Part model, mm, in its own coordinate system. Face numbers are marked on the shaded views. A direction names the side the tool comes from. Give positions to 0.01 mm unless a question says otherwise; leave off trailing zeros. Order: outer loops, then holes, each group sorted by start corner. A loop starts at its lowest first (then second) coordinate and runs counter-clockwise, first axis right, second up. Notation, with made-up numbers: (-33, -35) - (-27, -35) arc R27 cw to (-27, -3) - close; hole circle Ø2 at (-29.75, 15). An arc over 180 degrees is marked (long way). Use a Markdown table: item, result. Add a question column.
from build123d import *

# Parameters (mm, degrees)
SKETCH1_W           = 15.875
SKETCH1_H           = 44.45
BASE_EXTRUDE_DEPTH  = 22.225
SKETCH2_W           = 26.98496
SKETCH2_H           = 26.98496
BOSS_EXTRUDE1_DEPTH = 59.39536
SKETCH3_W           = 38.1
SKETCH3_H           = 38.1
BOSS_EXTRUDE2_DEPTH = 15.875
SKETCH4_R           = 2.09296
BOSS_EXTRUDE3_DEPTH = 59.39536
SKETCH5_R           = 1.45796
CUT_EXTRUDE1_DEPTH  = 75.27036
SKETCH6_R           = 4.7625
CUT_EXTRUDE2_DEPTH  = 75.27036
SKETCH8_R           = 3.175
CUT_EXTRUDE3_DEPTH  = 6.35


with BuildPart() as part:
    # Sketch1 → Base-Extrude (new, symmetric)
    with BuildSketch(Plane.XY):
        Rectangle(SKETCH1_W, SKETCH1_H)
    extrude(amount=BASE_EXTRUDE_DEPTH, both=True)

    # Sketch2 → Boss-Extrude1 (add)
    with BuildSketch(Plane(origin=(7.9375, 0, 0), x_dir=(0, 0, -1), z_dir=(1, 0, 0))):
        Rectangle(SKETCH2_W, SKETCH2_H)
    extrude(amount=BOSS_EXTRUDE1_DEPTH)

    # Sketch3 → Boss-Extrude2 (add)
    with BuildSketch(Plane(origin=(67.33286, -2.916482086, 3.369055623), x_dir=(0, 0, -1), z_dir=(1, 0, 0))):
        with Locations((3.369055623, 2.916482086)):
            Rectangle(SKETCH3_W, SKETCH3_H)
    extrude(amount=BOSS_EXTRUDE2_DEPTH)

    # Sketch4 → Boss-Extrude3 (add)
    with BuildSketch(Plane(origin=(7.9375, 0, 0), x_dir=(0, 0, -1), z_dir=(1, 0, 0))):
        with Locations((-13.49248, 13.49248)):
            Circle(SKETCH4_R)
        with Locations((-13.49248, -13.49248)):
            Circle(SKETCH4_R)
        with Locations((13.49248, 13.49248)):
            Circle(SKETCH4_R)
        with Locations((13.49248, -13.49248)):
            Circle(SKETCH4_R)
    extrude(amount=BOSS_EXTRUDE3_DEPTH)

    # Sketch5 → Cut-Extrude1 (cut)
    with BuildSketch(Plane(origin=(83.20786, 0, 0), x_dir=(0, 0, -1), z_dir=(1, 0, 0))):
        with Locations((-13.49248, 13.49248)):
            Circle(SKETCH5_R)
        with Locations((-13.49248, -13.49248)):
            Circle(SKETCH5_R)
        with Locations((13.49248, 13.49248)):
            Circle(SKETCH5_R)
        with Locations((13.49248, -13.49248)):
            Circle(SKETCH5_R)
    extrude(amount=-CUT_EXTRUDE1_DEPTH, mode=Mode.SUBTRACT)

    # Sketch6 → Cut-Extrude2 (cut)
    with BuildSketch(Plane.ZY.offset(7.9375)):
        Circle(SKETCH6_R)
    extrude(amount=-CUT_EXTRUDE2_DEPTH, mode=Mode.SUBTRACT)

    # Sketch8 → Cut-Extrude3 (cut)
    with BuildSketch(Plane.XY.offset(22.225)):
        Circle(SKETCH8_R)
    cut_extrude3 = extrude(amount=-CUT_EXTRUDE3_DEPTH, mode=Mode.SUBTRACT)

    # Mirror1: Cut-Extrude3 across plane
    add(cut_extrude3.mirror(Plane.XY), mode=Mode.SUBTRACT)


solid = part.part
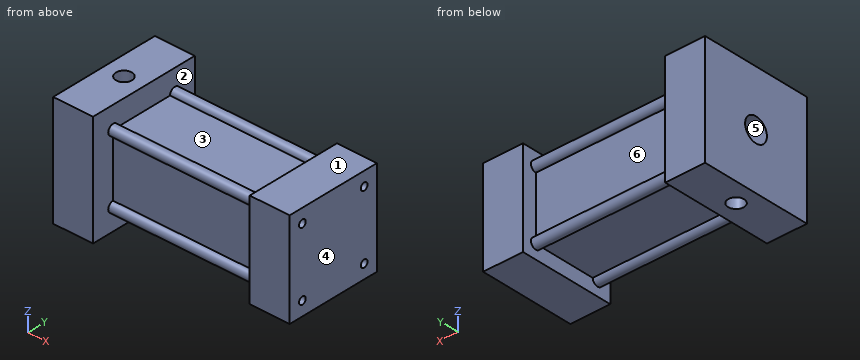
1. Cut at C-C (x = 75). Write the cut outline in (y, z).
2. Cut at A-A (x = 0). Write the cut outline in (y, z) (1 decimal), plus the area to 3 significant figures.
3. Mould opens along X. For the marked faces 4, 5 and 6 say: released by +X, released by -X, zero draft, split by the parting line, or undercut.
4. Drill centre lines: probe 1 along X at (y, z) = (14.5, -18); probe 2 along Z at (x, y) = (13.5, -15); probe 3 along Y at (x, z) = (39, -12.5). Where is each one in solid material? Low to high. Write a range as [from, to].
5. Pin check, flat tips, straight feed: P1, Ø7, axis at x = 51.5, z = 3.5, coming from the -Y side; P2, Ø1, axis at x = 40.5, z = 14.5, coming from the +Y side; P3, Ø5, axis at x = 0, y = 0, coming from the +Z side (3 decimals). Stop position of each tip, or through.
6. Tool access for the marked faces 1, 2 and 3: list every direction of +Z, -Z, +X, -X, +Y, -Y with a clear straight run to the whole face (end or side of a thin tool).
Responses:
| question | item | result |
|---|---|---|
| 1 | outline | (-19.05, -19.05) - (19.05, -19.05) - (19.05, 19.05) - (-19.05, 19.05) - close; hole circle Ø2.92 at (-13.49, -13.49); hole circle Ø2.92 at (-13.49, 13.49); hole circle Ø2.92 at (13.49, -13.49); hole circle Ø2.92 at (13.49, 13.49) |
| 2 | outline | (-22.2, -22.2) - (-3.2, -22.2) - (-3.2, -15.9) - (3.2, -15.9) - (3.2, -22.2) - (22.2, -22.2) - (22.2, 22.2) - (3.2, 22.2) - (3.2, 15.9) - (-3.2, 15.9) - (-3.2, 22.2) - (-22.2, 22.2) - close; hole circle Ø9.5 at (0, 0) |
| 2 | area | 1,820 mm² |
| 3 | face 4 | released by +X |
| 3 | face 5 | zero draft |
| 3 | face 6 | undercut |
| 4 | probe 1 | x = [-7.94, 7.94], [67.33, 83.21] |
| 4 | probe 2 | z = [-14.94, -12.04], [12.04, 14.94] |
| 4 | probe 3 | y = [-15.34, -14.56], [-12.42, 12.42], [14.56, 15.34] |
| 5 | P1 | stops at y = -13.49 |
| 5 | P2 | stops at y = 15.52 |
| 5 | P3 | stops at z = 15.875 |
| 6 | face 1 | +Z, +X, +Y, -Y |
| 6 | face 2 | none |
| 6 | face 3 | +Z |
